Could you check a few things on this model? Use its own coordinates, in mm. Face numbers are marked on the shaded views. A direction names the side the tool comes from. Coordinates: 2 decimals unless noted, no trailing zeros. Loops run counter-clockwise (first coordinate to the right, second up) from the corner with the lowest first, then second, coordinate; pieces in that order, holes last. Notation, with made-up numbers: M -4,-25.5 L 8,-25.5 A27 ccw 8,12.5 Z; hole C 18,44 d7. An arc over 180 degrees is marked long. Write each question's results on one line, items separated by ' | '.
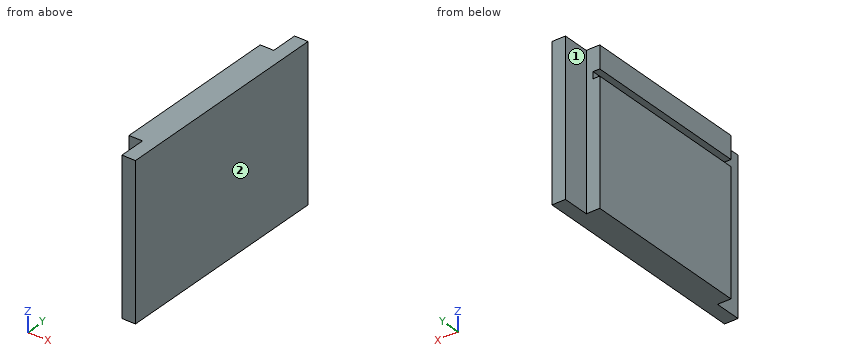
```python
from build123d import *

# Parameters (mm, degrees)
F1_DEPTH = 100
F3_DEPTH = 6
F5_DEPTH = 6


with BuildPart() as f1:
    # F0 (on Front) → F1 (new body)
    with BuildSketch(Plane.XZ):
        Polygon((-6, -34), (6, -34), (6, 34), (-6, 34), (-6, 24), (-3, 24), (-3, 21), (-6, 21), align=None)
    extrude(amount=F1_DEPTH)

    # F2 (on face) → F3 (cut)
    with BuildSketch(Plane(origin=(-6, 0, 0), x_dir=(0, -1, 0), z_dir=(-1, 0, 0))):
        Polygon((100.127715, -34), (100.127715, 34.181964), (88.127715, 34.181964), (88.107921, 34.181964), (88.107921, -34), align=None)
    extrude(amount=-F3_DEPTH, mode=Mode.SUBTRACT)

    # F4 (on face) → F5 (cut)
    with BuildSketch(Plane(origin=(-6, 0, 0), x_dir=(0, -1, 0), z_dir=(-1, 0, 0))):
        Polygon((12.064485, 34.181964), (0.814515, 34.181964), (0, 34.181964), (0, -34), (12.064485, -34), align=None)
    extrude(amount=-F5_DEPTH, mode=Mode.SUBTRACT)


solid = f1.part
```
(1) Which directions (+Z, -Z, +X, -X, +Y, -Y) give clear straight access to the entire face, cutting with the end or side of a thin tool? Please do the marked faces 1 and 2.
Reported:
face 1: +Z, -Z, -X, +Y | face 2: +Z, -Z, +X, +Y, -Y
(2) Will these pins go through, and if not, where does the flat tip stop? P1, Ø9.5, axis at y = -4, z = 1, coming from the -X side; P2, Ø1.8, axis at x = -4.5, z = 9.5, coming from the +Y side; P3, Ø6.5, axis at x = -4.5, z = 15.5, coming from the -Y side.
Reported:
P1: stops at x = 0 | P2: stops at y = -12.06 | P3: stops at y = -88.11
(3) Please list where these lines run through material, in increasing order: probe 1 along Z at (x, y) = (-4.25, -22); probe 2 along X at (y, z) = (-9, -21.5); probe 3 along Y at (x, z) = (-0.5, 0.5). Write a range as from..to.
Reported:
probe 1: z = -34..21, 24..34 | probe 2: x = 0..6 | probe 3: y = -88.11..-12.06
(4) Imagine slicing it at B-B, the plane z = 15.5. List the corners of the cut face in (x, y) for me, and give its area (3 significant figures).
Reported:
outline: M -6,-88.11 L 0,-88.11 L 0,-100 L 6,-100 L 6,0 L 0,0 L 0,-12.06 L -6,-12.06 Z | area: 1,060 mm2
(5) Imagine slicing it at A-A, the plane x = -4.5. List the corners of the cut face in (y, z) for me.
Reported:
outline: M -88.11,-34 L -12.06,-34 L -12.06,21 L -88.11,21 Z; M -88.11,24 L -12.06,24 L -12.06,34 L -88.11,34 Z
